Read the model definition and answer for the solid it produces. Units are mm, in the model's axes. Face numbers are marked on the shaded views. A direction names the side the tool comes from. Coordinates: 2 decimals unless noted, no trailing zeros. Order: outer loops, then holes, each group sorted by start corner. A loop starts at its lowest first (then second) coordinate and runs counter-clockwise, first axis right, second up. Notation, with made-up numbers: (80.5, 57.5) -> (91.5, 57.5) arc R19 ccw to (91.5, 77.5) -> close; hole circle Ø7 at (14, 72). An arc over 180 degrees is marked (long way). Return JSON: item names as keys, results as strings. Group by question number.
Autodesk Inventor part; units mm, degrees
ref_plane "YZ Plane" through (0, 0, 0) normal (1, 0, 0) x (0, 1, 0)
ref_plane "XZ Plane" through (0, 0, 0) normal (0, 1, 0) x (-1, 0, 0)
ref_plane "XY Plane" through (0, 0, 0) normal (0, 0, 1) x (1, 0, 0)
sketch "Sketch1" plane through (0, 0, 0) normal (0, 0, 1) x (1, 0, 0)
  line L0 (0, 0) -> (-10, 0)
  line L1 (-10, 0) -> (-10, 5)
  line L2 (-5, 10) -> (5, 10)
  line L3 (10, 5) -> (10, -5)
  line L4 (10, -5) -> (20, -5)
  line L5 (20, -5) -> (20, -10)
  line L6 (20, -10) -> (10, -10)
  line L7 (10, -10) -> (10, -15)
  line L8 (10, -15) -> (20, -15)
  line L9 (20, -15) -> (20, -17.9289)
  line L10 (18.5355, -21.4645) -> (11.4645, -28.5355)
  line L11 (7.9289, -30) -> (5, -30)
  line L12 (-10, -15) -> (-10, 0)
  arc A0 (-5, 10) -> (-10, 5) centre (-5, 5) ccw
  arc A1 (10, 5) -> (5, 10) centre (5, 5) ccw
  arc A2 (-10, -15) -> (5, -30) centre (5, -15) ccw
  arc A3 (7.9289, -30) -> (11.4645, -28.5355) centre (7.9289, -25) ccw
  arc A4 (18.5355, -21.4645) -> (20, -17.9289) centre (15, -17.9289) ccw
  line L13 (10, -10) -> (15, -10)
  line L14 (15, -10) -> (15, -15)
  point P0 (-10, 10)
  point P1 (10, 10)
  point P2 (20, -20)
  point P3 (10, -30)
  dimension "d0" = 10
  dimension "d1" = 10
  dimension "d2" = 20
  dimension "d3" = 15
  dimension "d4" = 10
  dimension "d5" = 5
  dimension "d6" = 5
  dimension "d7" = 5
  dimension "d8" = 135
  dimension "d9" = 5
  dimension "d10" = 15
  dimension "d11" = 5
  dimension "d21" = 5
extrude "Extrusion1" add sketch "Sketch1" along normal blind 5
sketch "Sketch2" plane through (0, 0, 5) normal (0, 0, 1) x (1, 0, 0)
  line L0 (0, 0) -> (0, 6)
  line L1 (0, 6) -> (5, 6)
  line L2 (5, 6) -> (-5, 6)
  circle A0 centre (-5, 6) radius 1.75
  circle A1 centre (5, 6) radius 1.75
  dimension "d14" = 6
  dimension "d15" = 5
  dimension "d16" = 10
  dimension "d17" = 3.5
  dimension "d18" = 3.5
extrude "Extrusion2" cut sketch "Sketch2" against normal blind 5
properties part number "holdBar"
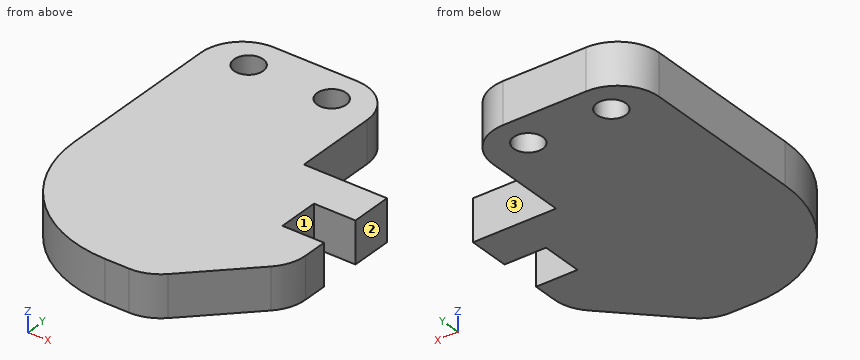
1. Straight lines are drawn through the part: L1, parallel to Y at x = 5, z = 2.5; L2, parallel to X at y = 7, z = 4; L3, parallel to X at y = 6.5, z = 0.35. For each, find the intervals that lie inside material, in ascending order.
2. Given pin 1 (3 mm diameter, centred on x = 13, y = -0.5, fed in from +Z); pin 2 (1.5 mm diameter, centred on y = -1, z = 1.5, fed in from +X); pin 3 (2.5 mm diameter, centred on x = 14, z = 2, fed in from +Y), each flat-ended and moving along its own axis, determine where each tip first touches the part or whether it passes through.
3. Find section A-A on y = 6. Determine the outline of the cut face in (x, z).
4. Find section B-B on z = 2.3. Determine the outline of the cut face in (x, y).
5. Find section C-C on x = -6. Determine the outline of the cut face in (y, z).
6. Which of the six approach directions +Z, -Z, +X, -X, +Y, -Y give full straight-line access (tool end or side, diameter ignored) to the marked faces 1, 2 and 3?
7. Find section D-D on x = 12.5. Determine the outline of the cut face in (y, z).
Result:
{
 "1": {"L1": "-30 to 4.25, 7.75 to 10", "L2": "-9.58 to -6.44, -3.56 to 3.56, 6.44 to 9.58", "L3": "-9.77 to -6.68, -3.32 to 3.32, 6.68 to 9.77"},
 "2": {"pin 1": "through", "pin 2": "x = 10", "pin 3": "y = -5"},
 "3": {"outline": "(-9.9, 0) -> (-6.75, 0) -> (-6.75, 5) -> (-9.9, 5) -> close; (-3.25, 0) -> (3.25, 0) -> (3.25, 5) -> (-3.25, 5) -> close; (6.75, 0) -> (9.9, 0) -> (9.9, 5) -> (6.75, 5) -> close"},
 "4": {"outline": "(-10, -15) arc R15 ccw to (5, -30) -> (7.93, -30) arc R5 ccw to (11.46, -28.54) -> (18.54, -21.46) arc R5 ccw to (20, -17.93) -> (20, -15) -> (15, -15) -> (15, -10) -> (20, -10) -> (20, -5) -> (10, -5) -> (10, 5) arc R5 ccw to (5, 10) -> (-5, 10) arc R5 ccw to (-10, 5) -> close; hole circle Ø3.5 at (-5, 6); hole circle Ø3.5 at (5, 6)"},
 "5": {"outline": "(-25.2, 0) -> (4.56, 0) -> (4.56, 5) -> (-25.2, 5) -> close; (7.44, 0) -> (9.9, 0) -> (9.9, 5) -> (7.44, 5) -> close"},
 "6": {"face 1": "+Z, -Z, +X", "face 2": "+Z, -Z, +X, +Y, -Y", "face 3": "+Z, -Z, +X, +Y"},
 "7": {"outline": "(-27.5, 0) -> (-5, 0) -> (-5, 5) -> (-27.5, 5) -> close"}
}
